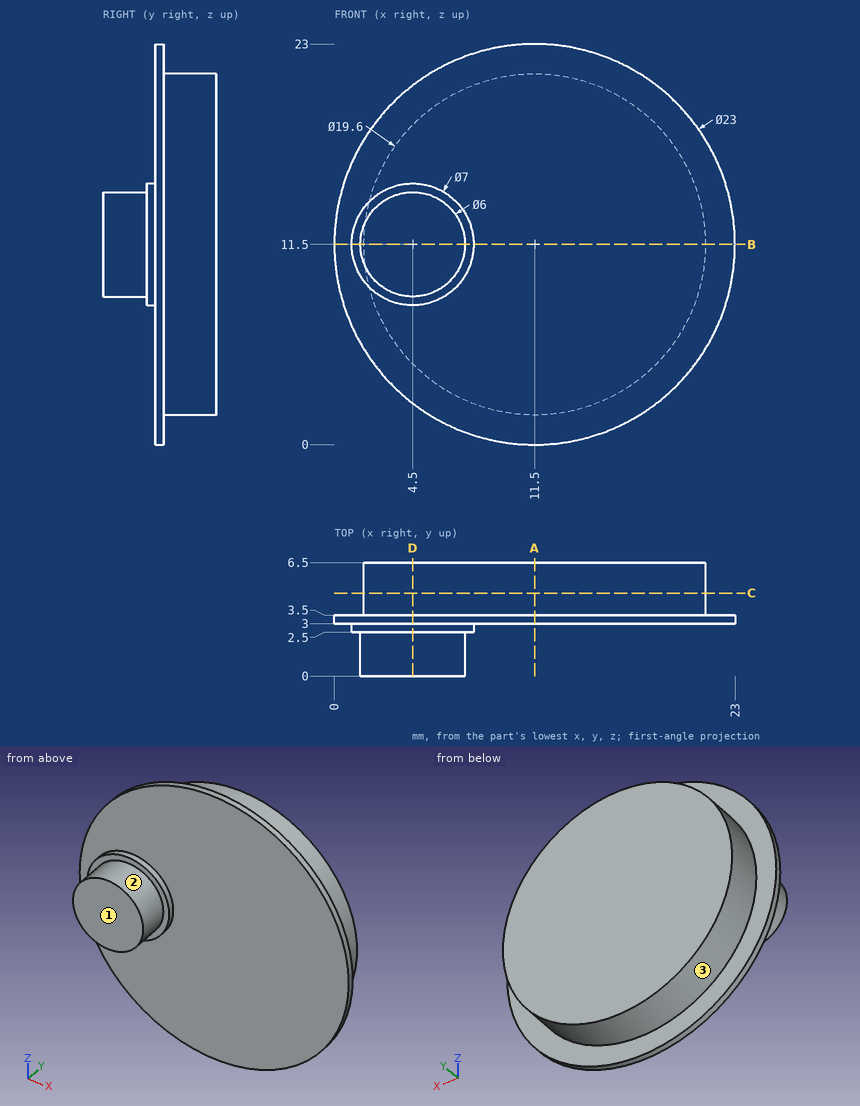
Input: dimensioned drawing with shaded views. Units: mm. Origin: part minimum x, y, z. A direction names the side the tool comes from. Give positions to 0.01 mm unless a question says otherwise; leave off trailing zeros. Write each loop counter-clockwise with the first axis right and the second up, starting at its lowest first coordinate (ties: lowest second). Pieces come first, ordered by that corner, then holes. Notation, with made-up numbers: (8, 45) - (55, 45) arc R17 ccw to (55, 49) - close; hole circle Ø4 at (76, 54.25). An arc over 180 degrees is marked (long way). One line per item, written item: value. Start each with the question number.
Q1. Material intervals for probe 1 along Y at (x, z) = (6, 4.5); probe 2 along Z at (x, y) = (4.5, 0.5); probe 3 along Z at (x, y) = (19.75, 3.25), sorted ascending. Write a range as from..to.
Q2. Section query A-A, the plane x = 11.5. Return the cut outline in (y, z), then the cut area to 3 significant figures.
Q3. Section query D-D, the plane x = 4.5. Return the cut outline in (y, z), then the cut area to 3 significant figures.
Q4. Section query B-B, the plane z = 11.5. Return the cut outline in (x, y).
Q5. Section query C-C, the plane y = 4.75. Return the cut outline in (x, z), then the cut area to 3 significant figures.
Q6. First-contact query: pin 1 Ø2 at (y, z) = (5.5, 17) entering from +X; pin 2 Ø12 at (x, z) = (12.5, 11.5) entering from -Y; pin 3 Ø3 at (x, y) = (9, 4.5) entering from +Z; pin 4 Ø6 at (x, z) = (14.5, 6) entering from -Y. Flat tips, straight axial feed; report the tip coordinate or a pass-through.
Q7. Set-up query: the marked faces 1, 2 and 3. Return all of +Z, -Z, +X, -X, +Y, -Y with unobstructed straight access to the full face (end or side cutting, diameter ignored); none if empty.
Answer:
1. probe 1: y = 3..6.5
1. probe 2: z = 8.5..14.5
1. probe 3: z = 3.49..19.51
2. outline: (3, 0) - (3.5, 0) - (3.5, 1.7) - (6.5, 1.7) - (6.5, 21.3) - (3.5, 21.3) - (3.5, 23) - (3, 23) - close
2. area: 70.3 mm2
3. outline: (0, 8.5) - (2.5, 8.5) - (2.5, 8) - (3, 8) - (3, 2.38) - (3.5, 2.38) - (3.5, 4.64) - (6.5, 4.64) - (6.5, 18.36) - (3.5, 18.36) - (3.5, 20.62) - (3, 20.62) - (3, 15) - (2.5, 15) - (2.5, 14.5) - (0, 14.5) - close
3. area: 68.8 mm2
4. outline: (0, 3) - (1, 3) - (1, 2.5) - (1.5, 2.5) - (1.5, 0) - (7.5, 0) - (7.5, 2.5) - (8, 2.5) - (8, 3) - (23, 3) - (23, 3.5) - (21.3, 3.5) - (21.3, 6.5) - (1.7, 6.5) - (1.7, 3.5) - (0, 3.5) - close
5. outline: circle Ø19.6 at (11.5, 11.5)
5. area: 302 mm2
6. pin 1: stops at x = 20.21
6. pin 2: stops at y = 0
6. pin 3: stops at z = 22.92
6. pin 4: stops at y = 3
7. face 1: +Z, -Z, +X, -X, -Y
7. face 2: -Y
7. face 3: +Y
